```python
from build123d import *

# Parameters (mm, degrees)
F1_DEPTH = 240
F2_R     = 2
F3_R     = 5


with BuildPart() as f1:
    # F0 (on Right) → F1 (new body)
    with BuildSketch(Plane.YZ):
        Polygon((-11.62, 7.9759603159), (-15.94, 12.2959603159), (-15.94, -0.5893383893), (-11.62, -0.5893383893), align=None)
        Polygon((-11.62, 11.0306616107), (-15.94, 15.3506616107), (-15.94, 12.2959603159), (-11.62, 7.9759603159), (-8.7938307864, 5.1497911023), (-7.266480139, 6.6771417497), align=None)
        Polygon((-8.5652987053, 11.0306616107), (-11.62, 11.0306616107), (-7.266480139, 6.6771417497), (-5.7391294917, 8.2044923971), align=None)
        Polygon((0, 15.3506616107), (-12.8852987053, 15.3506616107), (-8.5652987053, 11.0306616107), (0, 11.0306616107), align=None)
        Polygon((-12.8852987053, 15.3506616107), (-15.94, 15.3506616107), (-11.62, 11.0306616107), (-8.5652987053, 11.0306616107), align=None)
        Polygon((-15.94, -21.5946370946), (-11.62, -17.2746370946), (-11.62, -8.7093383893), (-15.94, -8.7093383893), align=None)
        Polygon((-3.625, -12.3343383893), (-3.625, -9.2796370946), (-11.62, -17.2746370946), (-15.94, -21.5946370946), (-15.94, -24.6493383893), (-12.8852987053, -24.6493383893), (-8.5652987053, -20.3293383893), (-0.5702987053, -12.3343383893), align=None)
        Polygon((0, -20.3293383893), (-8.5652987053, -20.3293383893), (-12.8852987053, -24.6493383893), (0, -24.6493383893), align=None)
        Polygon((14.9650698751, 9.3104327805), (8.6902987053, 3.0356616107), (11.745, 3.0356616107), (11.745, -0.0190396841), (18.0197711699, 6.2557314858), (19.74, 7.9759603159), (16.6852987053, 11.0306616107), align=None)
        Polygon((21.0052987053, 15.3506616107), (16.6852987053, 11.0306616107), (19.74, 7.9759603159), (24.06, 12.2959603159), (24.06, 15.3506616107), align=None)
        Polygon((24.06, 12.2959603159), (19.74, 7.9759603159), (19.74, -0.5893383893), (24.06, -0.5893383893), align=None)
        Polygon((8.12, 11.0306616107), (16.6852987053, 11.0306616107), (21.0052987053, 15.3506616107), (8.12, 15.3506616107), align=None)
        with BuildLine():
            Line((11.745, -9.2796370946), (11.745, -0.0190396841))
            Line((11.745, -0.0190396841), (7.4440143218, -4.3200253623))
            ThreePointArc((7.4440143218, -4.3200253623), (7.456001229, -4.4844879937), (7.46, -4.6493383893))
            ThreePointArc((7.46, -4.6493383893), (7.456001229, -4.8141887849), (7.4440143218, -4.9786514164))
            Line((7.4440143218, -4.9786514164), (11.745, -9.2796370946))
        make_face()
        with BuildLine():
            Line((3.7306869729, -8.0333527111), (-0.5702987053, -12.3343383893))
            Line((-0.5702987053, -12.3343383893), (8.6902987053, -12.3343383893))
            Line((8.6902987053, -12.3343383893), (4.3893130271, -8.0333527111))
            ThreePointArc((4.3893130271, -8.0333527111), (4.06, -8.0493383893), (3.7306869729, -8.0333527111))
        make_face()
        with BuildLine():
            Line((0.6759856782, -4.3200253623), (-3.625, -0.0190396841))
            Line((-3.625, -0.0190396841), (-3.625, -9.2796370946))
            Line((-3.625, -9.2796370946), (0.6759856782, -4.9786514164))
            ThreePointArc((0.6759856782, -4.9786514164), (0.66, -4.6493383893), (0.6759856782, -4.3200253623))
        make_face()
        with BuildLine():
            Line((8.6902987053, 3.0356616107), (-0.5702987053, 3.0356616107))
            Line((-0.5702987053, 3.0356616107), (3.7306869729, -1.2653240675))
            ThreePointArc((3.7306869729, -1.2653240675), (4.06, -1.2493383893), (4.3893130271, -1.2653240675))
            Line((4.3893130271, -1.2653240675), (8.6902987053, 3.0356616107))
        make_face()
        Polygon((-5.7391294917, 8.2044923971), (-7.266480139, 6.6771417497), (-3.625, 3.0356616107), (-0.5702987053, 3.0356616107), align=None)
        Polygon((-3.625, 3.0356616107), (-7.266480139, 6.6771417497), (-8.7938307864, 5.1497911023), (-3.625, -0.0190396841), align=None)
        Polygon((11.745, -12.3343383893), (8.6902987053, -12.3343383893), (16.6852987053, -20.3293383893), (21.0052987053, -24.6493383893), (24.06, -24.6493383893), align=None)
        Polygon((19.74, -17.2746370946), (11.745, -9.2796370946), (11.745, -12.3343383893), (24.06, -24.6493383893), (24.06, -21.5946370946), align=None)
        Polygon((19.74, -8.7093383893), (19.74, -17.2746370946), (24.06, -21.5946370946), (24.06, -8.7093383893), align=None)
        Polygon((21.0052987053, -24.6493383893), (16.6852987053, -20.3293383893), (8.12, -20.3293383893), (8.12, -24.6493383893), align=None)
        with BuildLine():
            Line((11.745, 3.0356616107), (8.6902987053, 3.0356616107))
            Line((8.6902987053, 3.0356616107), (4.3893130271, -1.2653240675))
            ThreePointArc((4.3893130271, -1.2653240675), (6.464163056, -2.2451753333), (7.4440143218, -4.3200253623))
            Line((7.4440143218, -4.3200253623), (11.745, -0.0190396841))
            Line((11.745, -0.0190396841), (11.745, 3.0356616107))
        make_face()
        with BuildLine():
            Line((1.655836944, -2.2451753333), (-3.625, 3.0356616107))
            Line((-3.625, 3.0356616107), (-3.625, -0.0190396841))
            Line((-3.625, -0.0190396841), (0.6759856782, -4.3200253623))
            ThreePointArc((0.6759856782, -4.3200253623), (0.9855894874, -3.1974430763), (1.655836944, -2.2451753333))
        make_face()
        with BuildLine():
            Line((0.6759856782, -4.9786514164), (-3.625, -9.2796370946))
            Line((-3.625, -9.2796370946), (-3.625, -12.3343383893))
            Line((-3.625, -12.3343383893), (-0.5702987053, -12.3343383893))
            Line((-0.5702987053, -12.3343383893), (3.7306869729, -8.0333527111))
            ThreePointArc((3.7306869729, -8.0333527111), (1.655836944, -7.0535014454), (0.6759856782, -4.9786514164))
        make_face()
        with BuildLine():
            Line((11.745, -12.3343383893), (6.464163056, -7.0535014454))
            ThreePointArc((6.464163056, -7.0535014454), (5.511895313, -7.7237489019), (4.3893130271, -8.0333527111))
            Line((4.3893130271, -8.0333527111), (8.6902987053, -12.3343383893))
            Line((8.6902987053, -12.3343383893), (11.745, -12.3343383893))
        make_face()
        with BuildLine():
            ThreePointArc((7.4440143218, -4.9786514164), (7.1344105126, -6.1012337024), (6.464163056, -7.0535014454))
            Line((6.464163056, -7.0535014454), (11.745, -12.3343383893))
            Line((11.745, -12.3343383893), (11.745, -9.2796370946))
            Line((11.745, -9.2796370946), (7.4440143218, -4.9786514164))
        make_face()
        with BuildLine():
            Line((-0.5702987053, 3.0356616107), (-3.625, 3.0356616107))
            Line((-3.625, 3.0356616107), (1.655836944, -2.2451753333))
            ThreePointArc((1.655836944, -2.2451753333), (2.608104687, -1.5749278767), (3.7306869729, -1.2653240675))
            Line((3.7306869729, -1.2653240675), (-0.5702987053, 3.0356616107))
        make_face()
    extrude(amount=F1_DEPTH)

    # F2
    f2_edges = [f1.edges().sort_by_distance(p)[0] for p in [
        (120, 0, 11.030662),
        (120, -11.62, -0.589338),
        (120, -15.94, -0.589338),
        (120, 0, 15.350662),
        (120, 8.12, 11.030662),
        (120, 19.74, -0.589338),
        (120, 24.06, -0.589338),
        (120, 8.12, -24.649338),
        (120, 8.12, 15.350662),
        (120, -15.94, -8.709338),
        (120, -11.62, -8.709338),
        (120, 0, -24.649338),
        (120, 0, -20.329338),
        (120, 8.12, -20.329338),
        (120, 19.74, -8.709338),
        (120, 24.06, -8.709338),
    ]]
    fillet(f2_edges, radius=F2_R)

    # F3
    f3_edges = [f1.edges().sort_by_distance(p)[0] for p in [
        (120, -15.94, 15.350662),
        (120, 24.06, 15.350662),
        (120, 24.06, -24.649338),
        (120, -15.94, -24.649338),
    ]]
    fillet(f3_edges, radius=F3_R)


solid = f1.part
```
Work out the finished part from the listing and answer in its coordinate system (mm). Give positions to 0.01 mm unless a question says otherwise; leave off trailing zeros. Loops run counter-clockwise (first coordinate to the right, second up) from the corner with the lowest first, then second, coordinate; pieces in that order, holes last. Notation, with made-up numbers: (-19, 47) -> (25, 47) arc R22 cw to (25, 58) -> close; hole circle Ø4 at (-13.5, 23). An arc over 180 degrees is marked (long way). Put each result on its own line as item: value. Start each with the question number.
Item 1: The mould has two halves that part along Y. Classify faces 1 (the face through (121.68, -14.51, -23.15)), 2 (the face through (118, 24.06, 6)), 3 (the face through (118.32, -7.567, -13.221)), 4 (the face through (118, -7, -24.649)): released by +Y, released by -Y, zero draft, split by the parting line, or undercut.
Item 2: Find the intervals of material crossed by L1, parallel to Z at x = 11.5, y = 15; L2, parallel to Y at x = 77.5, z = -14; L3, parallel to Y at x = 212, z = -4 (3 decimals), in increasing order. Write a range as [from, to].
Item 3: Each of these flat-tipped pins is pushed along its axis until it touches: P1, Ø10, axis at x = 156, z = -4, coming from the +Y side; P2, Ø5, axis at x = 62, z = -6.5, coming from the -Y side; P3, Ø4.5, axis at x = 124, z = -6, coming from the -Y side (3 decimals). Where does it stop, or does it pass through?
Item 4: The part is cut by section B-B (z = 5.5). Give the vertices of the cut face in (x, y), then the cut area to 3 significant figures.
Item 5: The part is cut by section A-A (y = -6). Give the vertices of the cut face in (x, z), then the cut area to 3 significant figures.
Answers below:
1. face 1: released by -Y
1. face 2: released by +Y
1. face 3: undercut
1. face 4: zero draft
2. L1: [-24.65, -20.33], [-18.64, -12.53], [3.24, 9.35], [11.03, 15.35]
2. L2: [-15.94, -11.62], [-8.35, -2.24], [10.36, 16.47], [19.74, 24.06]
2. L3: [-3.625, 0.723], [7.397, 11.745]
3. P1: y = 24.02
3. P2: y = -14.98
3. P3: y = -3.625
4. outline: (0, -15.94) -> (240, -15.94) -> (240, -11.62) -> (0, -11.62) -> close; (0, -9.14) -> (240, -9.14) -> (240, -3.03) -> (0, -3.03) -> close; (0, 11.15) -> (240, 11.15) -> (240, 17.26) -> (0, 17.26) -> close; (0, 19.74) -> (240, 19.74) -> (240, 24.06) -> (0, 24.06) -> close
4. area: 5,010 mm2
5. outline: (0, -24.65) -> (240, -24.65) -> (240, -20.33) -> (0, -20.33) -> close; (0, -17.76) -> (240, -17.76) -> (240, -11.65) -> (0, -11.65) -> close; (0, 2.36) -> (240, 2.36) -> (240, 8.47) -> (0, 8.47) -> close; (0, 11.03) -> (240, 11.03) -> (240, 15.35) -> (0, 15.35) -> close
5. area: 5,010 mm2
